```python
from build123d import *

# Parameters (mm, degrees)
F1_DEPTH = 9.525
F3_DEPTH = 9.525
F5_DEPTH = 25.4
F6_R     = 3.302
F7_DEPTH = 3.175


# Not quite as in the source:
# - a pattern or mirror of a feature is missing from the dataset's text; its kind, count and spacing are read off the source's solid


with BuildPart() as f1:
    # F0 (on Top) → F1 (new body)
    with BuildSketch(Plane.XY):
        Polygon((38.1, 0), (0, 38.1), (0, -38.1), align=None)
    extrude(amount=F1_DEPTH)

    # F2 (on face) → F3 (join)
    with BuildSketch(Plane.XY.offset(9.525)):
        with BuildLine():
            ThreePointArc((0, -38.1), (38.1, 0), (0, 38.1))
            Line((0, 38.1), (0, -38.1))
        make_face()
    extrude(amount=F3_DEPTH)

    # F4 (on face) → F5 (cut)
    with BuildSketch(Plane(origin=(0, 0, 0), x_dir=(1, 0, 0), z_dir=(0, 0, -1))):
        Polygon((9.525, 0), (0, 9.525), (0, -9.525), align=None)
    extrude(amount=-F5_DEPTH, mode=Mode.SUBTRACT)

    # F6 (on face) → F7 (cut)
    with BuildSketch(Plane(origin=(0, 0, 9.525), x_dir=(1, 0, 0), z_dir=(0, 0, -1))):
        with Locations((21.59, 21.59)):
            Circle(F6_R)
    f7 = extrude(amount=-F7_DEPTH, mode=Mode.SUBTRACT)

    # F7_copies: F7 across plane
    add(f7.mirror(Plane.ZX), mode=Mode.SUBTRACT)


solid = f1.part
```
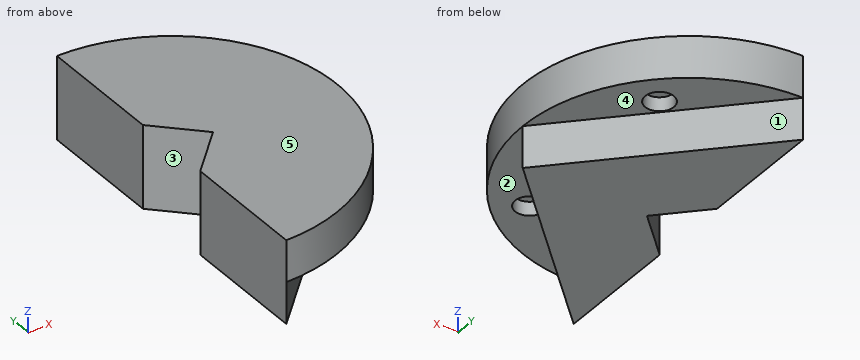
Part model, mm, in its own coordinate system. Face numbers are marked on the shaded views. A direction names the side the tool comes from. Coordinates: 2 decimals unless noted, no trailing zeros. Loops run counter-clockwise (first coordinate to the right, second up) from the corner with the lowest first, then second, coordinate; pieces in that order, holes last. Notation, with made-up numbers: (78, 5.5) - (131, 5.5) arc R27 ccw to (131, 29.5) - close; hole circle Ø4 at (37, 85.25). An arc over 180 degrees is marked (long way). Write item = value, one per line. Start each with the question number.
Item 1: Cut at C-C, the plane y = 33. Give the cut face in (x, z) (3 decimals), and give its area (3 significant figures).
Item 2: Wall check: L1, parallel to Y at x = 21.59, z = 12; L2, parallel to Z at x = 24.5, y = 23; L3, parallel to Y at x = 5, z = 13.25 (1 decimal). Give the ranges that are in metal, low to high. Write a range as from..to.
Item 3: Cut at A-A, the plane x = 3.5. Give the cut face in (y, z) (3 decimals).
Item 4: 3-axis set-ups, long thin cutter, end or side, ignore diameter. For the marked faces 4 and 5: which of +Z, -Z, +X, -X, +Y, -Y reach the whole face in a straight line?
Item 5: Cut at D-D, the plane x = 30.5. Give the cut face in (y, z) (3 decimals), and give its area (3 significant figures).
Item 6: Mould opens along Y. For the marked faces 1, 2 and 3 say: released by +Y, released by -Y, zero draft, split by the parting line, or undercut.
Item 7: Cut at B-B, the plane z = 16.25. Give the cut face in (x, y) (3 decimals).
Item 8: Flat gauge pins, fed straight in: pin 1 Ø3.5 at (x, y) = (23, -21.5) entering from -Z; pin 2 Ø3 at (x, z) = (13, 2.5) entering from +Y; pin 3 Ø6 at (x, z) = (8.5, 17) entering from -Y. Where does each tip first touch, or does it go through?
The answers:
q1.outline = (0, 0) - (5.1, 0) - (5.1, 9.525) - (19.042, 9.525) - (19.042, 19.05) - (0, 19.05) - close
q1.area = 230 mm2
q2.L1 = -31.39..-24.89, -18.29..18.29, 24.89..31.39
q2.L2 = 12.7..19.05
q2.L3 = -37.8..-4.5, 4.5..37.8
q3.outline = (-37.939, 9.525) - (-34.6, 9.525) - (-34.6, 0) - (-6.025, 0) - (-6.025, 19.05) - (-37.939, 19.05) - close; (6.025, 0) - (34.6, 0) - (34.6, 9.525) - (37.939, 9.525) - (37.939, 19.05) - (6.025, 19.05) - close
q4.face_4 = -Z, +X, +Y
q4.face_5 = +Z, +X, -X, +Y, -Y
q5.outline = (-22.833, 9.525) - (-7.6, 9.525) - (-7.6, 0) - (7.6, 0) - (7.6, 9.525) - (22.833, 9.525) - (22.833, 19.05) - (-22.833, 19.05) - close
q5.area = 580 mm2
q6.face_1 = released by +Y
q6.face_2 = zero draft
q6.face_3 = undercut
q7.outline = (0, -38.1) arc R38.1 ccw to (0, 38.1) - (0, 9.525) - (9.525, 0) - (0, -9.525) - close
q8.pin_1 = 12.7
q8.pin_2 = 26.6
q8.pin_3 = -37.7
